from build123d import *

# Parameters (mm, degrees)
SKETCH1_R           = 3.81
BOSS_EXTRUDE1_DEPTH = 19.05
SKETCH1_3_R         = 3.81
SKETCH1_3_R_2       = 2.159
BOSS_EXTRUDE2_DEPTH = 2.54
SKETCH2_W           = 6.35
SKETCH2_H           = 1.778
CUT_EXTRUDE2_DEPTH  = 35.29


with BuildPart() as part:
    # Sketch1 → Boss-Extrude1 (new body)
    with BuildSketch(Plane(origin=(0, 0, 0), x_dir=(1, 0, 0), z_dir=(0, 1, 0))):
        Polygon((-12.294680851, 17.581843972), (-31.344680851, 17.581843972), (-31.344680851, -16.708156028), (-12.294680851, -16.708156028), (-12.294680851, -12.898156028), (-5.944680851, -12.898156028), (-5.944680851, -16.708156028), (19.455319149, -16.708156028), (19.455319149, -12.898156028), (25.805319149, -12.898156028), (25.805319149, -16.708156028), (44.855319149, -16.708156028), (44.855319149, 17.581843972), (25.805319149, 17.581843972), (25.805319149, 13.771843972), (19.455319149, 13.771843972), (19.455319149, 17.581843972), (9.930319149, 17.581843972), (9.930319149, 4.881843972), (3.580319149, 4.881843972), (3.580319149, 17.581843972), (-5.944680851, 17.581843972), (-5.944680851, 13.771843972), (-12.294680851, 13.771843972), align=None)
        with Locations((-26.264680851, -11.628156028)):
            Circle(SKETCH1_R, mode=Mode.SUBTRACT)
        with Locations((39.775319149, -11.628156028)):
            Circle(SKETCH1_R, mode=Mode.SUBTRACT)
        with Locations((-26.264680851, 12.501843972)):
            Circle(SKETCH1_R, mode=Mode.SUBTRACT)
        with Locations((39.775319149, 12.501843972)):
            Circle(SKETCH1_R, mode=Mode.SUBTRACT)
    extrude(amount=BOSS_EXTRUDE1_DEPTH)

    # Sketch1_3 → Boss-Extrude2 (add)
    with BuildSketch(Plane(origin=(0, 0, 0), x_dir=(1, 0, 0), z_dir=(0, 1, 0))):
        with Locations((-26.264680851, 12.501843972)):
            Circle(SKETCH1_3_R)
        with Locations((-26.264680851, 12.501843972)):
            Circle(SKETCH1_3_R_2, mode=Mode.SUBTRACT)
        with Locations((-26.264680851, -11.628156028)):
            Circle(SKETCH1_3_R)
        with Locations((-26.264680851, -11.628156028)):
            Circle(SKETCH1_3_R_2, mode=Mode.SUBTRACT)
        with Locations((39.775319149, 12.501843972)):
            Circle(SKETCH1_3_R)
        with Locations((39.775319149, 12.501843972)):
            Circle(SKETCH1_3_R_2, mode=Mode.SUBTRACT)
        with Locations((39.775319149, -11.628156028)):
            Circle(SKETCH1_3_R)
        with Locations((39.775319149, -11.628156028)):
            Circle(SKETCH1_3_R_2, mode=Mode.SUBTRACT)
    extrude(amount=BOSS_EXTRUDE2_DEPTH)

    # Sketch2 → Cut-Extrude2 (cut, through all)
    with BuildSketch(Plane.XY.offset(16.708156028)):
        with Locations((-9.119680851, 0.889)):
            Rectangle(SKETCH2_W, SKETCH2_H)
        with Locations((22.630319149, 0.889)):
            Rectangle(SKETCH2_W, SKETCH2_H)
    extrude(amount=-CUT_EXTRUDE2_DEPTH, mode=Mode.SUBTRACT)


solid = part.part
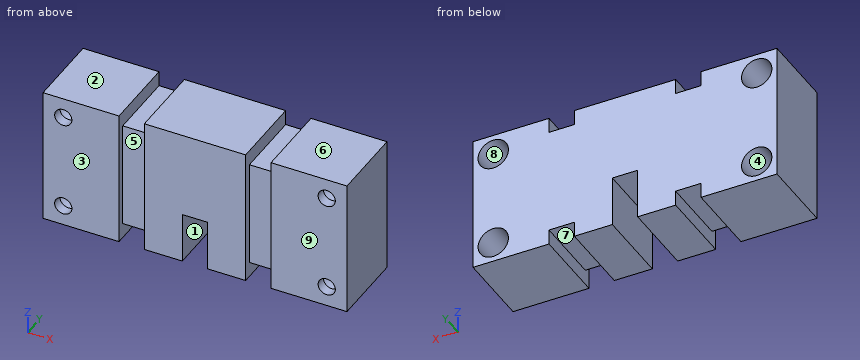
Could you check a few things on this model? Use its own coordinates, in mm. Face numbers are marked on the shaded views. A direction names the side the tool comes from. Coordinates: 2 decimals unless noted, no trailing zeros. Write each loop counter-clockwise with the first axis right and the second up, starting at its lowest first coordinate (ties: lowest second). Pieces come first, ordered by that corner, then holes. Notation, with made-up numbers: M 38,61.25 L 45,61.25 A16 ccw 45,68.25 Z; hole C 77.5,77.5 d7. An arc over 180 degrees is marked long. One line per question, with ' | ' between items.
1) I need wall thicknesses on probe 1 along X at (y, z) = (16.75, -8); probe 2 along X at (y, z) = (11.5, 10); probe 3 along X at (y, z) = (10, -16). Which ranges of each line are inside material? Lowest first, please. Write a range as [from, to].
Checks:
probe 1: [-31.34, 3.58], [9.93, 44.86] | probe 2: [-31.34, -29.71], [-22.82, 36.33], [43.22, 44.86] | probe 3: [-31.34, -27.77], [-24.76, -12.29], [-5.94, 3.58], [9.93, 19.46], [25.81, 38.27], [41.28, 44.86]
2) Imagine slicing it at A-A, the plane z = -7.5. Write out the boundary of the cut face in (x, y), and give its area (3 significant figures).
Checks:
outline: M -31.34,0 L -12.29,0 L -12.29,1.78 L -5.94,1.78 L -5.94,0 L 3.58,0 L 3.58,19.05 L -31.34,19.05 Z; M 9.93,0 L 19.46,0 L 19.46,1.78 L 25.81,1.78 L 25.81,0 L 44.86,0 L 44.86,19.05 L 9.93,19.05 Z | area: 1,310 mm²
3) Imagine slicing it at D-D, the plane x = 8.5. Write out the boundary of the cut face in (y, z).
Checks:
outline: M 0,-4.88 L 19.05,-4.88 L 19.05,16.71 L 0,16.71 Z
4) Imagine slicing it at B-B, the plane y = 11. Write out the boundary of the cut face in (x, z), and give its area (3 significant figures).
Checks:
outline: M -31.34,-17.58 L -12.29,-17.58 L -12.29,-13.77 L -5.94,-13.77 L -5.94,-17.58 L 3.58,-17.58 L 3.58,-4.88 L 9.93,-4.88 L 9.93,-17.58 L 19.46,-17.58 L 19.46,-13.77 L 25.81,-13.77 L 25.81,-17.58 L 44.86,-17.58 L 44.86,16.71 L 25.81,16.71 L 25.81,12.9 L 19.46,12.9 L 19.46,16.71 L -5.94,16.71 L -5.94,12.9 L -12.29,12.9 L -12.29,16.71 L -31.34,16.71 Z; hole C -26.26,-12.5 d7.62; hole C -26.26,11.63 d7.62; hole C 39.78,-12.5 d7.62; hole C 39.78,11.63 d7.62 | area: 2,250 mm²
5) For pin 1 Ø2.5 at (x, z) = (39.78, 11.63) entering from -Y; pin 2 Ø4 at (x, z) = (-27, 11) entering from +Y; pin 3 Ø1.9 at (x, y) = (-9, 8.5) entering from -Z; pin 4 Ø1.9 at (x, y) = (6, 12) entering from -Z, each with a flat end and sliding along its axis, tell me the tip position at first contact or that it passes through.
Checks:
pin 1: through | pin 2: y = 2.54 | pin 3: z = -13.77 | pin 4: z = -4.88
6) For the marked faces 1, 2, 3, 4 and 5, which set-ups out of +Z, -Z, +X, -X, +Y, -Y let a thin tool reach every point of the face, with its end or its side?
Checks:
face 1: -Z, +Y, -Y | face 2: +Z, +X, -X, +Y, -Y | face 3: +Z, -Z, +X, -X, -Y | face 4: +Y | face 5: +Z, -Z, -Y
7) Imagine slicing it at C-C, the plane z = 2. Write out the boundary of the cut face in (x, y), and give its area (3 significant figures).
Checks:
outline: M -31.34,0 L -12.29,0 L -12.29,1.78 L -5.94,1.78 L -5.94,0 L 19.46,0 L 19.46,1.78 L 25.81,1.78 L 25.81,0 L 44.86,0 L 44.86,19.05 L -31.34,19.05 Z | area: 1,430 mm²
8) If we mould it in two halves opening along Z, with no side actions, what happens to the marked faces 6, 7, 8 and 9? For each: released by +Z, released by -Z, zero draft, split by the parting line, or undercut.
Checks:
face 6: released by +Z | face 7: released by -Z | face 8: undercut | face 9: zero draft
